from build123d import *

# Parameters (mm, degrees)
SKETCH_1_W          = 17.6
SKETCH_1_H          = 21.8
EXTRUDE_1_DEPTH     = 1.56
SKETCH_2_W          = 15.21
SKETCH_2_H          = 15.21
CUT_EXTRUDE_1_DEPTH = 0.5
SKETCH_3_W          = 6.65
SKETCH_3_H          = 1.56
EXTRUDE_2_DEPTH     = 25.58
SKETCH_4_W          = 6.65
SKETCH_4_H          = 1
EXTRUDE_3_DEPTH     = 12.88
SKETCH_5_W          = 6.65
SKETCH_5_H          = 1
EXTRUDE_4_DEPTH     = 5.58
CUT_EXTRUDE_2_REACH = 45.766
SKETCH_6_W          = 6.65
SKETCH_6_H          = 12.88
CUT_EXTRUDE_3_REACH = 39.197
SKETCH_7_W          = 6.65
SKETCH_7_H          = 4.58


with BuildPart() as part:
    # 草图1 → 凸台-拉伸1 (new body)
    with BuildSketch(Plane(origin=(0, 0, 0), x_dir=(1, 0, 0), z_dir=(0, 1, 0))):
        with Locations((0.972375691, -4.190607735)):
            Rectangle(SKETCH_1_W, SKETCH_1_H)
    extrude(amount=EXTRUDE_1_DEPTH)

    # 草图2 → 切除-拉伸1 (cut)
    with BuildSketch(Plane(origin=(0, 1.56, 0), x_dir=(1, 0, 0), z_dir=(0, 1, 0))):
        with Locations((0.967375691, -2.095607735)):
            Rectangle(SKETCH_2_W, SKETCH_2_H)
    extrude(amount=-CUT_EXTRUDE_1_DEPTH, mode=Mode.SUBTRACT)

    # 草图3 → 凸台-拉伸2 (add)
    with BuildSketch(Plane.XY.offset(15.090607735)):
        with Locations((0.972375691, 0.78)):
            Rectangle(SKETCH_3_W, SKETCH_3_H)
    extrude(amount=EXTRUDE_2_DEPTH)

    # 草图4 → 凸台-拉伸3 (add)
    with BuildSketch(Plane(origin=(0, 0, 0), x_dir=(1, 0, 0), z_dir=(0, 1, 0))):
        with Locations((0.972375691, -27.290607735)):
            Rectangle(SKETCH_4_W, SKETCH_4_H)
    extrude(amount=-EXTRUDE_3_DEPTH)

    # 草图5 → 凸台-拉伸4 (add)
    with BuildSketch(Plane(origin=(0, 0, 26.790607735), x_dir=(-1, 0, 0), z_dir=(0, 0, -1))):
        with Locations((-0.972375691, -7.8)):
            Rectangle(SKETCH_5_W, SKETCH_5_H)
    extrude(amount=EXTRUDE_4_DEPTH)

    # 草图6 → 切除-拉伸2 (cut, up to next)
    with BuildSketch(Plane.XZ, mode=Mode.PRIVATE) as cut_extrude_2_sk1:
        with Locations((0.972375691, 34.230607735)):
            Rectangle(SKETCH_6_W, SKETCH_6_H)
    cut_extrude_2_tool1 = extrude(cut_extrude_2_sk1.sketch, amount=-CUT_EXTRUDE_2_REACH, mode=Mode.PRIVATE) & part.part
    add(cut_extrude_2_tool1.solids().sort_by_distance((0.972376, 0, 34.230608))[0], mode=Mode.SUBTRACT)

    # 草图7 → 切除-拉伸3 (cut, up to next)
    with BuildSketch(Plane(origin=(0, 0, 26.790607735), x_dir=(-1, 0, 0), z_dir=(0, 0, -1)), mode=Mode.PRIVATE) as cut_extrude_3_sk1:
        with Locations((-0.972375691, -10.59)):
            Rectangle(SKETCH_7_W, SKETCH_7_H)
    cut_extrude_3_tool1 = extrude(cut_extrude_3_sk1.sketch, amount=-CUT_EXTRUDE_3_REACH, mode=Mode.PRIVATE) & part.part
    add(cut_extrude_3_tool1.solids().sort_by_distance((0.972376, -10.59, 26.790608))[0], mode=Mode.SUBTRACT)


solid = part.part
The listing builds one solid part. Answer for the finished solid, in the listing's coordinates (mm). A direction names the side the tool comes from. Round coordinates to 2 decimals unless told otherwise and drop trailing zeros. Order: outer loops, then holes, each group sorted by start corner. A loop starts at its lowest first (then second) coordinate and runs counter-clockwise, first axis right, second up. Notation, with made-up numbers: (62, 58.25) -> (117, 58.25) arc R22 ccw to (117, 87.25) -> close; hole circle Ø3 at (54, 5). An arc over 180 degrees is marked (long way). Put each result on its own line as item: value.
Q1. Determine the mould class of faces 4 (the flat face through (1, -3, 27.791)), 5 (the flat face through (1, 1.06, 2)), 6 (the flat face through (1, 0, 6)) for opening direction Z: pulls with the +Z half, pulls with the -Z half, needs draft (parallel to the pull), parting line crosses it, or undercut.
Results list:
face 4: pulls with the +Z half
face 5: undercut
face 6: needs draft
Q2. Consider line 1 along Y through (x, z) = (-0.5, 24); line 2 along Y through (x, z) = (6.5, 7.5); line 3 along Z through (x, y) = (0.5, -3.5). Determine where each line is inside the solid, lowest interval first.
Results list:
line 1: -8.3 to -7.3, 0 to 1.56
line 2: 0 to 1.06
line 3: 26.79 to 27.79
Q3. Which of the six approach directions +Z, -Z, +X, -X, +Y, -Y give full straight-line access (tool end or side, diameter ignored) to faces 1 (the flat face through (7, 1, 15.091)), 2 (the flat face through (1, -4, 26.791)), 3 (the flat face through (1, -8, 21.211))?
Results list:
face 1: +Z, +X, +Y, -Y
face 2: -Z, +X, -X
face 3: -Z, +X, -X, -Y
Q4. Section A-A, the plane z = -4 is taken. Write down the section's boundary in (x, y), and give its area (3 significant figures).
Results list:
outline: (-7.83, 0) -> (9.77, 0) -> (9.77, 1.56) -> (8.57, 1.56) -> (8.57, 1.06) -> (-6.64, 1.06) -> (-6.64, 1.56) -> (-7.83, 1.56) -> close
area: 19.9 mm^2
Q5. Section B-B, the plane x = 3.25 is taken. Write down the section's boundary in (y, z), and give its area (3 significant figures).
Results list:
outline: (-8.3, 21.21) -> (-7.3, 21.21) -> (-7.3, 26.79) -> (0, 26.79) -> (0, -6.71) -> (1.56, -6.71) -> (1.56, -5.51) -> (1.06, -5.51) -> (1.06, 9.7) -> (1.56, 9.7) -> (1.56, 27.79) -> (-8.3, 27.79) -> close
area: 60.1 mm^2
Q6. Section D-D, the plane x = -2.75 is taken. Write down the section's boundary in (y, z).
Results list:
outline: (0, -6.71) -> (1.56, -6.71) -> (1.56, -5.51) -> (1.06, -5.51) -> (1.06, 9.7) -> (1.56, 9.7) -> (1.56, 15.09) -> (0, 15.09) -> close
Q7. Section C-C, the plane y = -5.75 is taken. Write down the section's boundary in (x, z).
Results list:
outline: (-2.35, 26.79) -> (4.3, 26.79) -> (4.3, 27.79) -> (-2.35, 27.79) -> close
Q8. Each of these flat-tipped pins is pushed along its axis until it touches: P1, Ø0.5, axis at x = 6, y = 1, coming from the +Z side; P2, Ø10, axis at x = 7, z = 3.5, coming from the -Y side; P3, Ø2, axis at x = -4.5, y = -1.5, coming from the +Z side; P4, Ø3.5, axis at x = 2, y = -3.5, coming from the -Z side. Where does it stop, or does it pass through?
Results list:
P1: z = 15.09
P2: y = 0
P3: through
P4: z = 26.79
